```python
from build123d import *

# Parameters (mm, degrees)
BOSS_EXTRUDE1_DEPTH      = 52.5
BOSS_EXTRUDE1_DEPTH_BACK = 52.5
CUT_EXTRUDE1_DEPTH       = 205.08331632
SKETCH3_W                = 90
SKETCH3_H                = 30
CUT_EXTRUDE2_DEPTH       = 205.08331632
CUT_EXTRUDE3_REACH       = 184.705
BOSS_EXTRUDE2_DEPTH      = 6.25


with BuildPart() as part:
    # Sketch1 → Boss-Extrude1 (new, two sides: drawn at the far end of the back side and taken through both)
    with BuildSketch(Plane.XY.offset(-BOSS_EXTRUDE1_DEPTH_BACK)):
        Polygon((-105, 0), (105, 0), (105, 60), (80, 60), (80, 140), (-80, 140), (-80, 60), (-105, 60), align=None)
    extrude(amount=BOSS_EXTRUDE1_DEPTH + BOSS_EXTRUDE1_DEPTH_BACK)

    # Sketch2 → Cut-Extrude1 (cut, through all)
    with BuildSketch(Plane.XY.offset(52.5)):
        with BuildLine():
            Line((-45, 0), (45, 0))
            ThreePointArc((45, 0), (0, 45), (-45, 0))
        make_face()
    extrude(amount=-CUT_EXTRUDE1_DEPTH, mode=Mode.SUBTRACT)

    # Sketch3 → Cut-Extrude2 (cut, through all)
    with BuildSketch(Plane.XY.offset(52.5)):
        with Locations((0, 105)):
            Rectangle(SKETCH3_W, SKETCH3_H)
    extrude(amount=-CUT_EXTRUDE2_DEPTH, mode=Mode.SUBTRACT)

    # Sketch5 → Cut-Extrude3 (cut, up to next)
    with BuildSketch(Plane(origin=(0, 140, 0), x_dir=(1, 0, 0), z_dir=(0, 1, 0)), mode=Mode.PRIVATE) as cut_extrude3_sk1:
        with BuildLine():
            Line((-20, 52.5), (-20, 31.721443851))
            ThreePointArc((-20, 31.721443851), (-37.5, 0), (-20, -31.721443851))
            Line((-20, -31.721443851), (-20, -52.5))
            Line((-20, -52.5), (20, -52.5))
            Line((20, -52.5), (20, -31.721443851))
            ThreePointArc((20, -31.721443851), (37.5, 0), (20, 31.721443851))
            Line((20, 31.721443851), (20, 52.5))
            Line((20, 52.5), (-20, 52.5))
        make_face()
    cut_extrude3_tool1 = extrude(cut_extrude3_sk1.sketch, amount=-CUT_EXTRUDE3_REACH, mode=Mode.PRIVATE) & part.part
    add(cut_extrude3_tool1.solids().sort_by_distance((0, 140, 0))[0], mode=Mode.SUBTRACT)

    # Sketch6 → Boss-Extrude2 (add, symmetric)
    with BuildSketch(Plane.XY):
        Polygon((80, 140), (105, 60), (80, 60), align=None)
    boss_extrude2 = extrude(amount=BOSS_EXTRUDE2_DEPTH, both=True)

    # Mirror1: Boss-Extrude2 across plane
    add(boss_extrude2.mirror(Plane(origin=(0, 0, 0), x_dir=(0, 0, 1), z_dir=(1, 0, 0))))


solid = part.part
```
The listing builds one solid part. Answer for the finished solid, in the listing's coordinates (mm). A direction names the side the tool comes from. Coordinates: 2 decimals unless noted, no trailing zeros. Order: outer loops, then holes, each group sorted by start corner. A loop starts at its lowest first (then second) coordinate and runs counter-clockwise, first axis right, second up. Notation, with made-up numbers: M 61,47.5 L 70,47.5 A12 cw 70,64.5 Z; hole C -38,52 d3. An arc over 180 degrees is marked long. Answer as a JSON object with one key per item and string values. Group by question number.
1. Section D-D on x = -41 is taken. Write down the section's boundary in (y, z), then the cut area to 3 significant figures.
2. Section A-A on y = 19 is taken. Write down the section's boundary in (x, z).
3. Section C-C on z = -36.5 is taken. Write down the section's boundary in (x, y), then the cut area to 3 significant figures.
4. Flat-ended cylindrical pins translate along their axes: P1, Ø10, axis at y = 133.5, z = -37.5, coming from the +X side; P2, Ø12.5, axis at x = 87, z = -28.5, coming from the +Y side; P3, Ø1.5, axis at y = 72, z = 16, coming from the -X side. Find the tip coordinate at first contact, or state that the pin passes through.
5. Determine the mould class of faces 6 (the flat face through (-45, 105, 1)), 7 (the flat face through (20, 130, -42)), 8 (the flat face through (-50, 140, -1)) for opening direction Y: released by +Y, released by -Y, zero draft, split by the parting line, or undercut.
6. Section B-B on y = 80 is taken. Write down the section's boundary in (x, z).
7. A tool of negligible diameter and unlimited length cuts with its end or side. For faces 1 (the cylindrical face through (37.496, 130.14, 0.529)), 2 (the flat face through (93, 60, 29)), 3 (the flat face through (-92, 60, -30)), 4 (the flat face through (45, 105, 1)), 5 (the flat face through (-20, 130, 42)), from which of +Z, -Z, +X, -X, +Y, -Y can it reach the whole face along a straight path? Write none if from no direction.
8. Straight lines are drawn through the part: line 1 (X direction, y = 102.5, z = 19); line 2 (Z direction, x = 86, y = 62.5); line 3 (Y direction, x = -38, z = 19.5). For each, find the intervals that lie inside material, in ascending order.
Values follow:
{
 "1": {"outline": "M 18.55,-52.5 L 90,-52.5 L 90,52.5 L 18.55,52.5 Z; M 120,-52.5 L 140,-52.5 L 140,52.5 L 120,52.5 Z", "area": "9,600 mm2"},
 "2": {"outline": "M -105,-52.5 L -40.79,-52.5 L -40.79,52.5 L -105,52.5 Z; M 40.79,-52.5 L 105,-52.5 L 105,52.5 L 40.79,52.5 Z"},
 "3": {"outline": "M -105,0 L -45,0 A45 cw 45,0 L 105,0 L 105,60 L 80,60 L 80,140 L 20,140 L 20,120 L 45,120 L 45,90 L -45,90 L -45,120 L -20,120 L -20,140 L -80,140 L -80,60 L -105,60 Z", "area": "18,700 mm2"},
 "4": {"P1": "x = 80", "P2": "y = 60", "P3": "x = -80"},
 "5": {"face 6": "undercut", "face 7": "zero draft", "face 8": "released by +Y"},
 "6": {"outline": "M -98.75,-6.25 L -80,-6.25 L -80,-52.5 L 80,-52.5 L 80,-6.25 L 98.75,-6.25 L 98.75,6.25 L 80,6.25 L 80,52.5 L -80,52.5 L -80,6.25 L -98.75,6.25 Z"},
 "7": {"face 1": "+Y", "face 2": "+Z, +X, +Y", "face 3": "-Z, -X, +Y", "face 4": "+Z, -Z", "face 5": "+Z, -Z, +Y"},
 "8": {"line 1": "-80 to -45, 45 to 80", "line 2": "-6.25 to 6.25", "line 3": "24.1 to 90, 120 to 140"}
}
